Autodesk Inventor part; units mm, degrees
ref_plane "Hole Work Plane" through (-20, 0, 0) normal (1, 0, 0) x (0, 1, 0)
ref_plane "XZ Plane" through (0, 0, 0) normal (0, 1, 0) x (-1, 0, 0)
ref_plane "XY Plane" through (0, 0, 0) normal (0, 0, 1) x (1, 0, 0)
sketch "Body Cross Section" plane through (0, 0, 0) normal (0, 1, 0) x (-1, 0, 0)
  circle A0 centre (0, 0) radius 9.5
  arc A1 (4.05, 3.0996) -> (4.05, -3.0996) centre (0, 0) ccw
  line L0 (4.05, -3.0996) -> (4.05, 3.0996)
  dimension "d0" = 19
  dimension "d1" = 10.2
  dimension "d2" = 4.05
extrude "Body" add sketch "Body Cross Section" along normal mid plane 7
ref_plane "Hole Work Plane" through (-20, 0, 0) normal (1, 0, 0) x (0, 1, 0)
sketch "Cable Hole Position" plane through (-20, 0, 0) normal (1, 0, 0) x (0, 1, 0)
  point P0 (0, 0)
  point P1 (0, 0)
hole "Cable Hole" at (-20, 0, 0) direction (1, 0, 0) diameter 3 end up to surface
fillet "Internal Fillet" radius 3.15 2 edges at (-4.05, 0, -3.0996) (-4.05, 0, 3.0996)
chamfer "Safety Chamfer" distance 0.5 angle 45 10 edges at (-3.5928, 3.5, 3.3643) (5.1, 3.5, 0) (-3.5928, 3.5, -3.3643) (-4.05, 3.5, 0) (5.1, -3.5, 0) (-3.5928, -3.5, -3.3643) (-4.05, -3.5, 0) (-3.5928, -3.5, 3.3643) (9.5, 3.5, 0) (9.5, -3.5, 0)
properties part number "Spacer" material "Aluminum 6061"
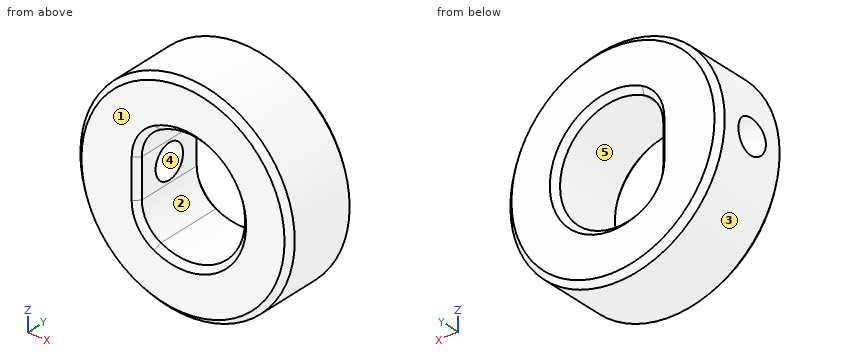
Build history of the part. All positions in model axes, mm. Face numbers are marked on the shaded views. A direction names the side the tool comes from. Round coordinates to 2 decimals unless told otherwise and drop trailing zeros. Write each loop counter-clockwise with the first axis right and the second up, starting at its lowest first coordinate (ties: lowest second). Pieces come first, ordered by that corner, then holes.
1) Pin check, flat tips, straight feed: pin 1 (8 mm diameter, centred on x = 0, z = 0, fed in from -Y); pin 2 (4 mm diameter, centred on x = 1, y = 2, fed in from +Z); pin 3 (1.5 mm diameter, centred on y = 1.5, z = -1.5, fed in from +X); pin 4 (1.5 mm diameter, centred on x = -7.5, y = -1.5, fed in from -Z). Stop position of each tip, or through.
2) Band-saw the part on D-D, the plane y = 0. List the corners of the cut face in (x, z), and give its area (3 significant figures).
3) Mould opens along X. For the marked faces 3, 4 and 5 say: +X half, -X half, draft (parallel to the pull), parting line (faces both ways), or undercut.
4) 3-axis set-ups, long thin cutter, end or side, ignore diameter. For the marked faces 1 and 2: which of +Z, -Z, +X, -X, +Y, -Y reach the whole face in a straight line?
5) Band-saw the part on C-C, the plane y = -2.5. List the corners of the cut face in (x, z).
6) Band-saw the part on B-B, the plane z = 0. List the corners of the cut face in (x, y), and give its area (3 significant figures).
7) Band-saw the part on A-A, the plane x = 0. List the corners of the cut face in (y, z), and give its area (3 significant figures).
8) Drill centre lines: probe 1 along Z at (x, y) = (0, -0.15); probe 2 along Y at (x, z) = (-7.8, 0); probe 3 along Z at (x, y) = (-5.2, 0). Where is each one in solid material? Low to high.
Ans:
1. pin 1: passes through
1. pin 2: stops at z = 9.5
1. pin 3: stops at x = 9.47
1. pin 4: stops at z = -6.68
2. outline: (-9.38, -1.5) arc R9.5 ccw (long way) to (-9.38, 1.5) - (-4.05, 1.5) - (-4.05, 1.73) arc R3.15 cw to (-2.35, 4.52) arc R5.1 cw (long way) to (-2.35, -4.52) arc R3.15 cw to (-4.05, -1.73) - (-4.05, -1.5) - close
2. area: 191 mm2
3. face 3: parting line
3. face 4: draft
3. face 5: undercut
4. face 1: +Z, -Z, +X, -X, -Y
4. face 2: +Y, -Y
5. outline: circle Ø19 at (0, 0); hole (-4.05, -1.73) arc R3.15 ccw to (-2.35, -4.52) arc R5.1 ccw (long way) to (-2.35, 4.52) arc R3.15 ccw to (-4.05, 1.73) - close
6. outline: (-9.5, -3) - (-9, -3.5) - (-4.55, -3.5) - (-4.05, -3) - (-4.05, -1.5) - (-9.5, -1.5) - close; (-9.5, 1.5) - (-4.05, 1.5) - (-4.05, 3) - (-4.55, 3.5) - (-9, 3.5) - (-9.5, 3) - close; (5.1, -3) - (5.6, -3.5) - (9, -3.5) - (9.5, -3) - (9.5, 3) - (9, 3.5) - (5.6, 3.5) - (5.1, 3) - close
6. area: 51.6 mm2
7. outline: (-3.5, -9) - (-3, -9.5) - (3, -9.5) - (3.5, -9) - (3.5, -5.6) - (3, -5.1) - (-3, -5.1) - (-3.5, -5.6) - close; (-3.5, 5.6) - (-3, 5.1) - (3, 5.1) - (3.5, 5.6) - (3.5, 9) - (3, 9.5) - (-3, 9.5) - (-3.5, 9) - close
7. area: 60.6 mm2
8. probe 1: z = -9.5 to -5.1, 5.1 to 9.5
8. probe 2: y = -3.5 to -1.5, 1.5 to 3.5
8. probe 3: z = -7.95 to -1.5, 1.5 to 7.95
